Here's how the part is built. I have some questions about the finished solid (model axes, mm). A direction names the side the tool comes from. Coordinates: 2 decimals unless noted, no trailing zeros. Order: outer loops, then holes, each group sorted by start corner. A loop starts at its lowest first (then second) coordinate and runs counter-clockwise, first axis right, second up. Notation, with made-up numbers: (13.25, 73.25) - (61.25, 73.25) arc R19 ccw to (61.25, 100.25) - close; hole circle Ø7 at (2, -34.75). An arc over 180 degrees is marked (long way). Answer as CSV lines item,"result". Start each with the question number.
Q1. Suppose I cut it at D-D (x = 7.5). Please give me the cut outline in (y, z).
Q2. I need wall thicknesses on line 1 (Y direction, x = 96, z = 1.4); line 2 (X direction, y = -0.75, z = 1.75); line 3 (Y direction, x = 77.5, z = 4.75). Which ranges of each line are inside material? Lowest first, please.
Q3. Suppose I cut it at B-B (z = 1). Please give me the cut outline in (x, y).
Q4. Thinking about a two-plate mould opening in Y: for faces 4 (the face through (93, 6, 3)), 5 (the face through (93, 0, 3)), 6 (the face through (7.2, -5.77, 2.96)), which applies, released by +Y, released by -Y, zero draft, split by the parting line, or undercut?
Q5. Suppose I cut it at A-A (y = 0). Please give me the cut outline in (x, z), then the cut area to 3 significant figures.
Q6. For pin 1 Ø5.5 at (x, y) = (0, 0) entering from +Z; pin 2 Ø3 at (x, z) = (49.5, 1.5) entering from -Y; pin 3 Ø2 at (y, z) = (5, 1.5) entering from -X, each with a flat end and sliding along its axis, tell me the tip position at first contact or that it passes through.
Q7. Suppose I cut it at C-C (x = 36.5). Please give me the cut outline in (y, z), then the cut area to 3 significant figures.
Q8. For faces 1 (the face through (11.65, 4.23, 2.96)), 2 (the face through (102, 0, 3)), 3 (the face through (88.745, -5.756, 3.042)), which set-ups out of +Z, -Z, +X, -X, +Y, -Y let a thin tool reach every point of the face, with its end or its side?
from build123d import *

# Parameters (mm, degrees)
SKETCH1_R           = 3
BOSS_EXTRUDE2_DEPTH = 6
SKETCH2_W           = 60
SKETCH2_H           = 4
CUT_EXTRUDE2_DEPTH  = 103.352332655
CHAMFER2_SIZE       = 10.722534603
CHAMFER2_SIZE_2     = 5
FILLET2_R           = 10


with BuildPart() as part:
    # Sketch1 → Boss-Extrude2 (new body)
    with BuildSketch(Plane.XY):
        with BuildLine():
            Line((0, 6), (96, 6))
            ThreePointArc((96, 6), (102, 0), (96, -6))
            Line((96, -6), (0, -6))
            ThreePointArc((0, -6), (-6, 0), (0, 6))
        make_face()
        Circle(SKETCH1_R, mode=Mode.SUBTRACT)
        with Locations((96, 0)):
            Circle(SKETCH1_R, mode=Mode.SUBTRACT)
    extrude(amount=BOSS_EXTRUDE2_DEPTH)

    # Sketch2 → Cut-Extrude2 (cut, through all)
    with BuildSketch(Plane.XY.offset(6)):
        with Locations((48, -6)):
            Rectangle(SKETCH2_W, SKETCH2_H)
        with Locations((48, 6)):
            Rectangle(SKETCH2_W, SKETCH2_H)
    extrude(amount=-CUT_EXTRUDE2_DEPTH, mode=Mode.SUBTRACT)

    # Chamfer2
    # the kernel refuses this chamfer: 10.722534603, 5 mm, written as the material it takes off along each edge
    with BuildSketch(Plane(origin=(78, 6, -27.781824147), x_dir=(0.9998669641130703, 0.01631116413111023, 0), z_dir=(0, 0, 1))) as chamfer2_piece_1_section:
        Polygon((CHAMFER2_SIZE * 0.999866964071, -CHAMFER2_SIZE * 0.0163111641304), (-CHAMFER2_SIZE_2 * 0.0163111641311, -CHAMFER2_SIZE_2 * 0.999866964113), (0, 0), align=None)
    chamfer2_piece_1 = extrude(amount=61.563648293, mode=Mode.PRIVATE)
    chamfer2_piece_1 = split(chamfer2_piece_1, bisect_by=Plane(origin=(82.533411446, 4, 3), z_dir=(0, 1, 0)), keep=Keep.TOP, mode=Mode.PRIVATE)
    add(chamfer2_piece_1, mode=Mode.SUBTRACT)
    with BuildSketch(Plane(origin=(78, -6, -27.781824147), x_dir=(-0.07481330637060442, 0.997197557753677, 0), z_dir=(0, 0, 1))) as chamfer2_piece_2_section:
        Polygon((CHAMFER2_SIZE_2 * 0.997197557754, -CHAMFER2_SIZE_2 * 0.0748133063706), (-CHAMFER2_SIZE * 0.0748133063675, -CHAMFER2_SIZE * 0.997197557712), (0, 0), align=None)
    chamfer2_piece_2 = extrude(amount=61.563648293, mode=Mode.PRIVATE)
    chamfer2_piece_2 = split(chamfer2_piece_2, bisect_by=Plane(origin=(82.533411446, -4, 3), z_dir=(0, -1, 0)), keep=Keep.TOP, mode=Mode.PRIVATE)
    add(chamfer2_piece_2, mode=Mode.SUBTRACT)
    with BuildSketch(Plane(origin=(18, -6, 33.781824147), x_dir=(-0.9998669641130703, -0.0163111641311102, 0), z_dir=(0, 0, -1))) as chamfer2_piece_3_section:
        Polygon((CHAMFER2_SIZE * 0.999866964071, CHAMFER2_SIZE * 0.0163111641304), (-CHAMFER2_SIZE_2 * 0.0163111641311, CHAMFER2_SIZE_2 * 0.999866964113), (0, 0), align=None)
    chamfer2_piece_3 = extrude(amount=61.563648293, mode=Mode.PRIVATE)
    chamfer2_piece_3 = split(chamfer2_piece_3, bisect_by=Plane(origin=(13.466588554, -4, 3), z_dir=(0, -1, 0)), keep=Keep.TOP, mode=Mode.PRIVATE)
    add(chamfer2_piece_3, mode=Mode.SUBTRACT)
    with BuildSketch(Plane(origin=(18, 6, 33.781824147), x_dir=(-0.9998669641130703, 0.016311164131110195, 0), z_dir=(0, 0, -1))) as chamfer2_piece_4_section:
        Polygon((CHAMFER2_SIZE * 0.999866964071, -CHAMFER2_SIZE * 0.0163111641304), (-CHAMFER2_SIZE_2 * 0.0163111641311, -CHAMFER2_SIZE_2 * 0.999866964113), (0, 0), align=None)
    chamfer2_piece_4 = extrude(amount=61.563648293, mode=Mode.PRIVATE)
    chamfer2_piece_4 = split(chamfer2_piece_4, bisect_by=Plane(origin=(13.466588554, 4, 3), z_dir=(0, 1, 0)), keep=Keep.TOP, mode=Mode.PRIVATE)
    add(chamfer2_piece_4, mode=Mode.SUBTRACT)

    # Fillet2
    fillet2_edges = [part.edges().sort_by_distance(p)[0] for p in [
        (88.722534603, 6, 3),
        (88.722534603, -6, 3),
        (7.277465397, -6, 3),
        (7.277465397, 6, 3),
        (84.433520762, 4, 3),
        (84.433520762, -4, 3),
        (11.566479238, -4, 3),
        (11.566479238, 4, 3),
    ]]
    fillet(fillet2_edges, radius=FILLET2_R)


solid = part.part
Here are the results:
1,outline,"(-5.7, 0) - (5.7, 0) - (5.7, 6) - (-5.7, 6) - close"
2,line 1,"y = -6 to -3, 3 to 6"
2,line 2,"x = -5.95 to -2.9, 2.9 to 93.1, 98.9 to 101.95"
2,line 3,"y = -4 to 4"
3,outline,"(0, -6) - (5.06, -6) arc R10 ccw to (9.29, -5.06) - (9.56, -4.94) arc R10 cw to (13.78, -4) - (82.22, -4) arc R10 cw to (86.44, -4.94) - (86.71, -5.06) arc R10 ccw to (90.94, -6) - (96, -6) arc R6 ccw to (96, 6) - (90.94, 6) arc R10 ccw to (86.71, 5.06) - (86.44, 4.94) arc R10 cw to (82.22, 4) - (13.78, 4) arc R10 cw to (9.56, 4.94) - (9.29, 5.06) arc R10 ccw to (5.06, 6) - (0, 6) arc R6 ccw to start; hole circle Ø6 at (0, 0); hole circle Ø6 at (96, 0)"
4,face 4,"released by +Y"
4,face 5,"undercut"
4,face 6,"released by -Y"
5,outline,"(-6, 0) - (-3, 0) - (-3, 6) - (-6, 6) - close; (3, 0) - (93, 0) - (93, 6) - (3, 6) - close; (99, 0) - (102, 0) - (102, 6) - (99, 6) - close"
5,area,"576 mm²"
6,pin 1,"passes through"
6,pin 2,"stops at y = -4"
6,pin 3,"stops at x = -4.47"
7,outline,"(-4, 0) - (4, 0) - (4, 6) - (-4, 6) - close"
7,area,"48.0 mm²"
8,face 1,"+Z, -Z, +Y"
8,face 2,"+Z, -Z, +X"
8,face 3,"+Z, -Z, -Y"
